Geometry check sheet. Reference: the model listing, model coordinates, mm. A direction names the side the tool comes from. Round coordinates to 2 decimals unless told otherwise and drop trailing zeros. Write each loop counter-clockwise with the first axis right and the second up, starting at its lowest first coordinate (ties: lowest second). Pieces come first, ordered by that corner, then holes. Notation, with made-up numbers: (79, 31.25) -> (117, 31.25) arc R30 cw to (117, 53.25) -> close; hole circle Ø3 at (7.25, -39.5). An arc over 180 degrees is marked (long way). Return JSON: item names as keys, results as strings. Group by question number.
from build123d import *

# Parameters (mm, degrees)
SKETCH_1_W        = 66
SKETCH_1_H        = 20
EXTRUDE_224_DEPTH = 1.5
EXTRUDE_START     = 1.5
SKETCH_2_W        = 1.5
SKETCH_2_H        = 20
EXTRUDE_307_DEPTH = 50.5
EXTRUDE_START_2   = 52
SKETCH_3_W        = 66
SKETCH_3_H        = 20
EXTRUDE_387_DEPTH = 1.5


with BuildPart() as part:
    # 草图1 → Extrude 224 (new body)
    with BuildSketch(Plane.XY):
        Rectangle(SKETCH_1_W, SKETCH_1_H)
    extrude(amount=EXTRUDE_224_DEPTH)

    # 草图2 → Extrude 307 (add)
    with BuildSketch(Plane.XY.offset(EXTRUDE_START)):
        with Locations((-32.25, 0)):
            Rectangle(SKETCH_2_W, SKETCH_2_H)
        with Locations((32.25, 0)):
            Rectangle(SKETCH_2_W, SKETCH_2_H)
    extrude(amount=EXTRUDE_307_DEPTH)

    # 草图3 → Extrude 387 (add)
    with BuildSketch(Plane.XY.offset(EXTRUDE_START_2)):
        Rectangle(SKETCH_3_W, SKETCH_3_H)
    extrude(amount=EXTRUDE_387_DEPTH)


solid = part.part
1) Sectioned sample at A-A on x = 8. Enter the section's corners in (y, z).
2) Sectioned sample at C-C on y = 4.75. Enter the section's corners in (x, z).
3) Tool access check on faces 1 (the face through (0, 0, 52)), 2 (the face through (-33, 0, 26)). Record the directions out of +Z, -Z, +X, -X, +Y, -Y that give a thin tool (end or side, any length) a straight path to the whole face; none if there is none.
4) Sectioned sample at B-B on z = 32.5. Enter the section's corners in (x, y).
5) Mould release check, pull along X, two halves, no side actions. Record for faces 3 (the face through (0, 0, 1.5)), 4 (the face through (33, 0, 26)), 5 (the face through (0, 0, 0)): +X half, -X half, draft (parallel to the pull), parting line (faces both ways), or undercut.
6) Material ranges on probe 1 along X at (y, z) = (0.5, 38); probe 2 along Z at (x, y) = (-20, -8.5), recorded low to high. Write a range as [from, to].
Evaluation:
{
 "1": {"outline": "(-10, 0) -> (10, 0) -> (10, 1.5) -> (-10, 1.5) -> close; (-10, 52) -> (10, 52) -> (10, 53.5) -> (-10, 53.5) -> close"},
 "2": {"outline": "(-33, 0) -> (33, 0) -> (33, 53.5) -> (-33, 53.5) -> close; hole (-31.5, 1.5) -> (31.5, 1.5) -> (31.5, 52) -> (-31.5, 52) -> close"},
 "3": {"face 1": "+Y, -Y", "face 2": "+Z, -Z, -X, +Y, -Y"},
 "4": {"outline": "(-33, -10) -> (-31.5, -10) -> (-31.5, 10) -> (-33, 10) -> close; (31.5, -10) -> (33, -10) -> (33, 10) -> (31.5, 10) -> close"},
 "5": {"face 3": "undercut", "face 4": "+X half", "face 5": "draft"},
 "6": {"probe 1": "x = [-33, -31.5], [31.5, 33]", "probe 2": "z = [0, 1.5], [52, 53.5]"}
}
